from build123d import *

# Parameters (mm, degrees)
EXTRUDE_1_DEPTH        = 100
SKETCH_2_R             = 30
CUT_EXTRUDE_1_DEPTH    = 100
SKETCH_3_R             = 32.5
SKETCH_3_R_2           = 30
EXTRUDE_2_DEPTH        = 5
EXTRUDE_START          = 5
SKETCH_4_R             = 32.5
SKETCH_4_R_2           = 30
EXTRUDE_3_DEPTH        = 5
SKETCH_5_R             = 30
CUT_EXTRUDE_3_DEPTH    = 552
SKETCH_6_R             = 35
SKETCH_6_R_2           = 30
EXTRUDE_4_DEPTH        = 5
SKETCH_7_R             = 35
SKETCH_7_R_2           = 30
EXTRUDE_5_DEPTH        = 5
SKETCH_8_R             = 50
EXTRUDE_6_DEPTH        = 448
EXTRUDE_7_DEPTH        = 10
SKETCH_10_R            = 30
CUT_EXTRUDE_4_DEPTH    = 10
PATTERN_LINEAR_1_COUNT = 2
PATTERN_LINEAR_1_PITCH = 80
MIRROR_2_COPY_1_DEPTH  = 10
SKETCH_11_R            = 30
CUT_EXTRUDE_5_DEPTH    = 800
SCALE1_SCALE           = 0.345


with BuildPart() as part:
    # 草图1 → 凸台-拉伸1 (new body)
    with BuildSketch(Plane.XY):
        with BuildLine():
            Line((-60.1323511, -127.533248731), (739.8676489, -277.533248731))
            Line((739.8676489, -277.533248731), (4439.8676489, -277.533248731))
            ThreePointArc((4439.8676489, -277.533248731), (4514.8676489, -202.533248731), (4439.8676489, -127.533248731))
            Line((4439.8676489, -127.533248731), (3639.8676489, 22.466751269))
            Line((3639.8676489, 22.466751269), (-60.1323511, 22.466751269))
            ThreePointArc((-60.1323511, 22.466751269), (-135.1323511, -52.533248731), (-60.1323511, -127.533248731))
        make_face()
    extrude(amount=EXTRUDE_1_DEPTH)

    # 草图2 → 切除-拉伸1 (cut)
    with BuildSketch(Plane.XY.offset(100)):
        with Locations((-60.1323511, -52.533248731)):
            Circle(SKETCH_2_R)
        with Locations((4439.8676489, -202.533248731)):
            Circle(SKETCH_2_R)
    extrude(amount=-CUT_EXTRUDE_1_DEPTH, mode=Mode.SUBTRACT)

    # 草图3 → 凸台-拉伸2 (add)
    # profile 1 of 2: a face of its own
    with BuildSketch(Plane(origin=(0, 0, 0), x_dir=(-1, 0, 0), z_dir=(0, 0, -1))):
        with Locations(Location((-4439.8676489, -202.533248731, 0), (0, 0, 180))):
            Circle(SKETCH_3_R)
        with Locations(Location((-4439.8676489, -202.533248731, 0), (0, 0, 180))):
            Circle(SKETCH_3_R_2, mode=Mode.SUBTRACT)
    # profile 2 of 2: a face of its own
    with BuildSketch(Plane(origin=(0, 0, 0), x_dir=(-1, 0, 0), z_dir=(0, 0, -1))):
        with Locations(Location((60.1323511, -52.533248731, 0), (0, 0, 180))):
            Circle(SKETCH_3_R)
        with Locations(Location((60.1323511, -52.533248731, 0), (0, 0, 180))):
            Circle(SKETCH_3_R_2, mode=Mode.SUBTRACT)
    extrude(amount=EXTRUDE_2_DEPTH)

    # 草图4 → 凸台-拉伸3 (add)
    # profile 1 of 2: a face of its own
    with BuildSketch(Plane.XY.offset(100).offset(EXTRUDE_START)):
        with Locations((-60.1323511, -52.533248731)):
            Circle(SKETCH_4_R)
        with Locations((-60.1323511, -52.533248731)):
            Circle(SKETCH_4_R_2, mode=Mode.SUBTRACT)
    # profile 2 of 2: a face of its own
    with BuildSketch(Plane.XY.offset(100).offset(EXTRUDE_START)):
        with Locations((4439.8676489, -202.533248731)):
            Circle(SKETCH_4_R)
        with Locations((4439.8676489, -202.533248731)):
            Circle(SKETCH_4_R_2, mode=Mode.SUBTRACT)
    extrude(amount=-EXTRUDE_3_DEPTH)

    # 草图5 → 切除-拉伸3 (cut)
    with BuildSketch(Plane(origin=(0, 0, 0), x_dir=(-1, 0, 0), z_dir=(0, 0, -1))):
        with Locations((-2189.8676489, -127.533248731)):
            Circle(SKETCH_5_R)
    extrude(amount=-CUT_EXTRUDE_3_DEPTH, mode=Mode.SUBTRACT)

    # 草图6 → 凸台-拉伸4 (add)
    with BuildSketch(Plane.XY.offset(100)):
        with Locations((2189.8676489, -127.533248731)):
            Circle(SKETCH_6_R)
        with Locations(Location((2189.8676489, -127.533248731, 0), (0, 0, 180))):
            Circle(SKETCH_6_R_2, mode=Mode.SUBTRACT)
    extrude(amount=EXTRUDE_4_DEPTH)

    # 草图7 → 凸台-拉伸5 (add)
    with BuildSketch(Plane(origin=(0, 0, 0), x_dir=(-1, 0, 0), z_dir=(0, 0, -1)).offset(EXTRUDE_START)):
        with Locations(Location((-2189.8676489, -127.533248731, 0), (0, 0, 180))):
            Circle(SKETCH_7_R)
        with Locations((-2189.8676489, -127.533248731)):
            Circle(SKETCH_7_R_2, mode=Mode.SUBTRACT)
    extrude(amount=-EXTRUDE_5_DEPTH)

    # 草图8 → 凸台-拉伸6 (add)
    with BuildSketch(Plane(origin=(0, 0, 0), x_dir=(-1, 0, 0), z_dir=(0, 0, -1))):
        with Locations(Location((-3175.422502192, -127.533248731, 0), (0, 0, 180))):
            Circle(SKETCH_8_R)
    extrude(amount=EXTRUDE_6_DEPTH)

    # 镜向1: part across plane


with BuildPart() as part_1:
    add(part.part)
    add(part.part.mirror(Plane(origin=(3175.422502192, -127.533248731, -448), x_dir=(1, 0, 0), z_dir=(0, 0, -1))))

    # 草图9 → 凸台-拉伸7 (add)
    with BuildSketch(Plane(origin=(0, 0, -736), x_dir=(-1, 0, 0), z_dir=(0, 0, -1))):
        with BuildLine():
            Line((-3006.157635441, -1.638829142), (-3196.193047707, -60.685777283))
            ThreePointArc((-3196.193047707, -60.685777283), (-3239.857841934, -154.884427725), (-3141.764888729, -188.91048438))
            Line((-3141.764888729, -188.91048438), (-2967.280379028, -93.22790564))
            ThreePointArc((-2967.280379028, -93.22790564), (-2945.296288829, -29.850466609), (-3006.157635441, -1.638829142))
        make_face()
    extrude_7 = extrude(amount=EXTRUDE_7_DEPTH)

    # 草图10 → 切除-拉伸4 (cut)
    with BuildSketch(Plane(origin=(0, 0, -746), x_dir=(-1, 0, 0), z_dir=(0, 0, -1))):
        with Locations((-2991.321531502, -49.387023033)):
            Circle(SKETCH_10_R)
    extrude(amount=-CUT_EXTRUDE_4_DEPTH, mode=Mode.SUBTRACT)

    # 阵列(线性)1: 凸台-拉伸7 ×2
    with Locations(*[(0, 0, -i * PATTERN_LINEAR_1_PITCH) for i in range(1, PATTERN_LINEAR_1_COUNT)]):
        add(extrude_7)

    # 镜向2: 凸台-拉伸7 across plane
    add(extrude_7.mirror(Plane(origin=(0, 0, -448), x_dir=(1, 0, 0), z_dir=(0, 0, -1))))

    # 镜向2 copy 1 sketch → 镜向2 copy 1 (add)
    with BuildSketch(Plane(origin=(0, 0, -80), x_dir=(-1, 0, 0), z_dir=(0, 0, 1))):
        with BuildLine():
            Line((-3006.157635441, 1.638829142), (-3196.193047707, 60.685777283))
            ThreePointArc((-3196.193047707, 60.685777283), (-3239.857841934, 154.884427725), (-3141.764888729, 188.91048438))
            Line((-3141.764888729, 188.91048438), (-2967.280379028, 93.22790564))
            ThreePointArc((-2967.280379028, 93.22790564), (-2945.296288829, 29.850466609), (-3006.157635441, 1.638829142))
        make_face()
    extrude(amount=MIRROR_2_COPY_1_DEPTH)

    # 草图11 → 切除-拉伸5 (cut)
    with BuildSketch(Plane(origin=(0, 0, -826), x_dir=(-1, 0, 0), z_dir=(0, 0, -1))):
        with Locations((-2991.321531502, -49.387023033)):
            Circle(SKETCH_11_R)
    extrude(amount=-CUT_EXTRUDE_5_DEPTH, mode=Mode.SUBTRACT)


with BuildPart() as part_2:
    # Scale1: scaled about (2220.490419966, -127.389558081, -448)
    add(part_1.part.scale(SCALE1_SCALE).moved(Location((1454.421225078, -83.440160543, -293.44))))


solid = part_2.part
Work out the finished part from the listing and answer in its coordinate system (mm). A direction names the side the tool comes from. Give positions to 0.01 mm unless a question says otherwise; leave off trailing zeros. Order: outer loops, then holes, each group sorted by start corner. A loop starts at its lowest first (then second) coordinate and runs counter-clockwise, first axis right, second up. Notation, with made-up numbers: (14, 30) -> (37, 30) arc R13 cw to (37, 44) -> close; hole circle Ø8 at (-19, -33). An arc over 180 degrees is marked (long way). One line per item, written item: value.
Item 1: Flat-ended cylindrical pins translate along their axes: P1, Ø16.5, axis at x = 2486.43, y = -100.48, coming from the +Z side; P2, Ø1, axis at x = 2740, y = -107, coming from the -Z side; P3, Ø12, axis at y = -111.5, z = -373, coming from the +X side. Find the tip coordinate at first contact, or state that the pin passes through.
Answer sheet:
P1: z = -258.94
P2: z = -637.06
P3: x = 2564.04
Item 2: Find section B-B, the plane z = -280. Give the vertices of the cut face in (x, y) (3 decimals).
Answer sheet:
outline: (1433.676, -127.439) -> (1709.676, -179.189) -> (2986.176, -179.189) arc R25.875 ccw to (2986.176, -127.439) -> (2710.176, -75.689) -> (1433.676, -75.689) arc R25.875 ccw to start; hole circle Ø20.7 at (1433.676, -101.564); hole circle Ø20.7 at (2209.926, -127.439); hole circle Ø20.7 at (2986.176, -153.314)
Item 3: Find section A-A, the plane x = 2788.5. Give the vertices of the cut face in (y, z).
Answer sheet:
outline: (-179.19, -637.06) -> (-90.37, -637.06) -> (-90.37, -602.56) -> (-179.19, -602.56) -> close; (-179.19, -293.44) -> (-90.37, -293.44) -> (-90.37, -258.94) -> (-179.19, -258.94) -> close
Item 4: A tool of negligible diameter and unlimited length cuts with its end or side. For faces 1 (the flat face through (2081, -75.689, -620)), 2 (the cylindrical face through (2566.4, -132.6, -305.3)), 3 (the flat face through (2508.65, -132.34, -319.34)), from which of +Z, -Z, +X, -X, +Y, -Y can it reach the whole face along a straight path? Write none if from no direction.
Answer sheet:
face 1: +Z, -Z, +X, -X, +Y
face 2: none
face 3: -X, -Y
Item 5: Determine the mould class of faces 4 (the flat face through (2081, -75.689, -276)), 5 (the flat face through (2199, -115, -637.06)), 6 (the flat face through (2522, -117, -348.64)), 7 (the cylindrical face through (2566.4, -132.6, -563.1)) for opening direction Z: released by +Z, released by -Z, zero draft, split by the parting line, or undercut.
Answer sheet:
face 4: zero draft
face 5: released by -Z
face 6: undercut
face 7: undercut
Item 6: Straight lines are drawn through the part: probe 1 along Z at (x, y) = (1608.5, -122); probe 2 along X at (y, z) = (-148.5, -601.5); probe 3 along X at (y, z) = (-142.5, -524.5). For each, find the intervals that lie inside material, in ascending order.
Answer sheet:
probe 1: -637.06 to -602.56, -293.44 to -258.94
probe 2: 2976.05 to 2977.01, 2995.34 to 2996.3
probe 3: 2541.53 to 2558.35
Item 7: Find section C-C, the plane x = 1750.5. Give the vertices of the cut face in (y, z), plus the area to 3 significant figures.
Answer sheet:
outline: (-179.19, -637.06) -> (-75.69, -637.06) -> (-75.69, -602.56) -> (-179.19, -602.56) -> close; (-179.19, -293.44) -> (-75.69, -293.44) -> (-75.69, -258.94) -> (-179.19, -258.94) -> close
area: 7,140 mm²
Item 8: Find section D-D, the plane z = -376.5. Give the vertices of the cut face in (x, y), plus the area to 3 significant figures.
Answer sheet:
outline: circle Ø34.5 at (2549.94, -127.44)
area: 935 mm²
